from build123d import *

# Parameters (mm, degrees)
SKETCH1_R               = 60
BOSS_EXTRUDE1_DEPTH     = 5
SKETCH2_W               = 92
SKETCH2_H               = 66
CUT_EXTRUDE1_DEPTH      = 4.5
SKETCH3_W               = 66
SKETCH3_H               = 18.4
CUT_EXTRUDE2_DEPTH      = 4.5
CUT_EXTRUDE3_DEPTH      = 5.5
CUT_EXTRUDE3_DEPTH_BACK = 1.5
BOSS_EXTRUDE4_DEPTH     = 66
BOSS_EXTRUDE5_DEPTH     = 66
LPATTERN1_COUNT         = 5
LPATTERN1_PITCH         = 18.8
SKETCH10_R              = 1.905
CUT_EXTRUDE4_DEPTH      = 6
SKETCH11_W              = 1.982288408
SKETCH11_H              = 73.369538915
CUT_EXTRUDE5_DEPTH      = 4.5
LPATTERN2_COUNT         = 4
LPATTERN2_PITCH         = 18.8
SKETCH12_R              = 1.905
CUT_EXTRUDE6_DEPTH      = 6


with BuildPart() as part:
    # Sketch1 → Boss-Extrude1 (new body)
    with BuildSketch(Plane.XY):
        Circle(SKETCH1_R)
    extrude(amount=BOSS_EXTRUDE1_DEPTH)

    # Sketch2 → Cut-Extrude1 (cut)
    with BuildSketch(Plane.XY.offset(5)):
        with Locations((0, 5)):
            Rectangle(SKETCH2_W, SKETCH2_H)
    extrude(amount=-CUT_EXTRUDE1_DEPTH, mode=Mode.SUBTRACT)

    # Sketch3 → Cut-Extrude2 (cut)
    with BuildSketch(Plane.XY.offset(5)):
        with Locations((0, -38.2)):
            Rectangle(SKETCH3_W, SKETCH3_H)
    extrude(amount=-CUT_EXTRUDE2_DEPTH, mode=Mode.SUBTRACT)

    # Sketch4 → Cut-Extrude3 (cut, two sides)
    with BuildSketch(Plane.XY.offset(0.5)) as cut_extrude3_sk:
        with BuildLine():
            Line((-38.173943993, 43), (38.173943993, 43))
            ThreePointArc((38.173943993, 43), (0, 57.5), (-38.173943993, 43))
        make_face()
    extrude(amount=CUT_EXTRUDE3_DEPTH, mode=Mode.SUBTRACT)
    extrude(cut_extrude3_sk.sketch, amount=-CUT_EXTRUDE3_DEPTH_BACK, mode=Mode.SUBTRACT)

    # Sketch8 → Boss-Extrude4 (add)
    with BuildSketch(Plane(origin=(-33, 0, 0), x_dir=(0, 0, -1), z_dir=(1, 0, 0))):
        with BuildLine():
            Line((-5, -47.4), (-5, -46.187250507))
            ThreePointArc((-5, -46.187250507), (-2.139853595, -43.520930962), (-0.645401314, -39.907579367))
            Line((-0.645401314, -39.907579367), (-0.5, -39.907579367))
            Line((-0.5, -39.907579367), (-0.5, -47.4))
            Line((-0.5, -47.4), (-5, -47.4))
        make_face()
        with BuildLine():
            Line((-5, -29), (-5, -30.369538915))
            ThreePointArc((-5, -30.369538915), (-2.101750406, -33.091237194), (-0.622561202, -36.781696722))
            Line((-0.622561202, -36.781696722), (-0.5, -36.781696722))
            Line((-0.5, -36.781696722), (-0.5, -29))
            Line((-0.5, -29), (-5, -29))
        make_face()
    extrude(amount=BOSS_EXTRUDE4_DEPTH)

    # Sketch9 → Boss-Extrude5 (add)
    with BuildSketch(Plane(origin=(-30.969379717, 38, 37.672222409), x_dir=(0, 0, -1), z_dir=(0, -1, 0))):
        with BuildLine():
            Line((32.672222409, -15.030620283), (32.672222409, -14.530620283))
            ThreePointArc((32.672222409, -14.530620283), (35.383633316, -12.07254318), (36.922222409, -8.751905327))
            Line((36.922222409, -8.751905327), (37.172222409, -8.751905327))
            Line((37.172222409, -8.751905327), (37.172222409, -15.030620283))
            Line((37.172222409, -15.030620283), (32.672222409, -15.030620283))
        make_face()
        with BuildLine():
            Line((32.672222409, 1.787091309), (32.672222409, 1.287091309))
            ThreePointArc((32.672222409, 1.287091309), (35.383633316, -1.170985793), (36.922222409, -4.491623646))
            Line((36.922222409, -4.491623646), (37.172222409, -4.491623646))
            Line((37.172222409, -4.491623646), (37.172222409, 1.787091309))
            Line((37.172222409, 1.787091309), (32.672222409, 1.787091309))
        make_face()
    boss_extrude5 = extrude(amount=BOSS_EXTRUDE5_DEPTH)

    # LPattern1: Boss-Extrude5 ×5
    with Locations(*[(i * LPATTERN1_PITCH, 0, 0) for i in range(1, LPATTERN1_COUNT)]):
        add(boss_extrude5)

    # Sketch10 → Cut-Extrude4 (cut, through all)
    with BuildSketch(Plane(origin=(0, 0, 0), x_dir=(-1, 0, 0), z_dir=(0, 0, -1))):
        with Locations((-52.017711592, 0)):
            Circle(SKETCH10_R)
        with Locations((51.982288408, 0)):
            Circle(SKETCH10_R)
    extrude(amount=-CUT_EXTRUDE4_DEPTH, mode=Mode.SUBTRACT)

    # Sketch11 → Cut-Extrude5 (cut)
    with BuildSketch(Plane.XY.offset(5)):
        with Locations((-28.191144204, 6.315230542)):
            Rectangle(SKETCH11_W, SKETCH11_H)
    cut_extrude5 = extrude(amount=-CUT_EXTRUDE5_DEPTH, mode=Mode.SUBTRACT)

    # LPattern2: Cut-Extrude5 ×4
    with Locations(*[(i * LPATTERN2_PITCH, 0, 0) for i in range(1, LPATTERN2_COUNT)]):
        add(cut_extrude5, mode=Mode.SUBTRACT)

    # Sketch12 → Cut-Extrude6 (cut, through all)
    with BuildSketch(Plane(origin=(0, 0, 0), x_dir=(-1, 0, 0), z_dir=(0, 0, -1))):
        with Locations((-50.654578855, 11.67355769)):
            Circle(SKETCH12_R)
        with Locations((-50.654578855, -11.67355769)):
            Circle(SKETCH12_R)
        with Locations((50.654578855, -11.67355769)):
            Circle(SKETCH12_R)
        with Locations((50.654578855, 11.67355769)):
            Circle(SKETCH12_R)
    extrude(amount=-CUT_EXTRUDE6_DEPTH, mode=Mode.SUBTRACT)


solid = part.part
Read the model definition and answer for the solid it produces. Units are mm, in the model's axes. A direction names the side the tool comes from. Give positions to 0.01 mm unless a question says otherwise; leave off trailing zeros. Write each loop counter-clockwise with the first axis right and the second up, starting at its lowest first coordinate (ties: lowest second). Pieces come first, ordered by that corner, then holes. Notation, with made-up numbers: (71.5, -35) - (121.5, -35) arc R23 ccw to (121.5, -13) - close; hole circle Ø9 at (32.5, -17). An arc over 180 degrees is marked (long way). Use CSV: the item, a comma, the result in double quotes. Start each with the question number.
(1) Determine the mould class of faces 1 (the flat face through (-1, 1, 0)), 2 (the flat face through (33, -38, 3)) for opening direction Y: +Y half, -Y half, draft (parallel to the pull), parting line (faces both ways), or undercut.
(2) Find section A-A (x = 0). Give the vertices of the cut face in (y, z).
(3) For faces 3 (the flat face through (19, -28, 3)), 4 (the flat face through (10.7, 11.9, 5)), determine the directions among +Z, -Z, +X, -X, +Y, -Y from which every point of the face is accessible in a straight line to the end or side of a thin tool.
(4) Find section D-D (x = -42). Give the vertices of the cut face in (y, z).
(5) Find section B-B (y = -44). Give the vertices of the cut face in (x, z), plus the area to 3 significant figures.
(6) Consider line 1 along X through (y, z) = (11.5, 0.35); line 2 along X through (y, z) = (41, 4); line 3 along Y through (x, z) = (-8, 2.5). Determine where each line is inside the solid, lowest interval first.
(7) Given P1, Ø2, axis at x = 36, z = 3, coming from the +Y side; P2, Ø0.6, axis at x = -9.5, z = 3, coming from the +Y side; P3, Ø1.3, axis at x = 0.5, z = 2.5, coming from the -Y side, each flat-ended and moving along its own axis, determine where each tip first touches the part or whether it passes through.
(8) Find section C-C (y = 0). Count the separate pieces of the cut face and the enclosed holes in it, plus the area to 3 significant figures.
Findings below:
1,face 1,"draft"
1,face 2,"undercut"
2,outline,"(-60, 0) - (43, 0) - (43, 5) - (38, 5) - (38, 0.5) - (-28, 0.5) - (-28, 5) - (-30.37, 5) arc R9.2 cw to (-36.78, 0.62) - (-36.78, 0.5) - (-39.91, 0.5) - (-39.91, 0.65) arc R9.2 cw to (-46.19, 5) - (-60, 5) - close; (57.5, 0) - (60, 0) - (60, 5) - (57.5, 5) - close"
3,face 3,"+Z"
3,face 4,"+Z, +X, -X, +Y, -Y"
4,outline,"(-42.85, 0) - (42.85, 0) - (42.85, 5) - (38, 5) - (38, 1.63) - (-28, 1.63) - (-28, 5) - (-42.85, 5) - close"
5,outline,"(-40.79, 0) - (40.79, 0) - (40.79, 5) - (33, 5) - (33, 2.5) - (-33, 2.5) - (-33, 5) - (-40.79, 5) - close"
5,area,"243 mm2"
6,line 1,"-58.89 to -52.55, -48.76 to 48.76, 52.55 to 58.89"
6,line 2,"-43.81 to -29.18, -27.2 to -10.38, -8.4 to 8.42, 10.4 to 27.22, 29.2 to 43.81"
6,line 3,"-59.46 to -44.01, -32.55 to 43, 56.94 to 59.46"
7,P1,"y = 48.73"
7,P2,"y = 59.29"
7,P3,"y = -60"
8,separate pieces,"3"
8,enclosed holes,"0"
8,area,"272 mm2"
